Part model, mm, in its own coordinate system. Coordinates: 2 decimals unless noted, no trailing zeros. Order: outer loops, then holes, each group sorted by start corner. A loop starts at its lowest first (then second) coordinate and runs counter-clockwise, first axis right, second up.
from build123d import *

# Parameters (mm, degrees)
F1_DEPTH = 4.253926
F2_R     = 2.54
F3_DEPTH = 4.16477


with BuildPart() as f1:
    # F0 (on Front) → F1 (new body, symmetric)
    with BuildSketch(Plane.XZ):
        Polygon((25.404785, 14.029387), (13.940861, 0), (13.940861, -34.714542), (45.487791, 0), (45.487791, 42.974394), (25.404785, 42.974394), align=None)
    extrude(amount=F1_DEPTH, both=True)

    # F2
    f2_edges = [f1.edges().sort_by_distance(p)[0] for p in [
        (19.672823, -4.253926, 7.014694),
        (13.940861, -4.253926, -17.357271),
        (29.714326, -4.253926, -17.357271),
        (45.487791, -4.253926, 21.487197),
        (35.446288, -4.253926, 42.974394),
        (25.404785, -4.253926, 28.501891),
    ]]
    fillet(f2_edges, radius=F2_R)

    # F1_face (on face) → F3 (join)
    with BuildSketch(Plane(origin=(31.070742, -4.253926, 8.875899), x_dir=(1, 0, 0), z_dir=(0, -1, 0))):
        Polygon((-3.125957, 4.247698), (-14.589881, -9.781689), (-14.589881, -37.01865), (11.87705, -7.894188), (11.87705, 31.558495), (-3.125957, 31.558495), align=None)
    extrude(amount=F3_DEPTH)


solid = f1.part
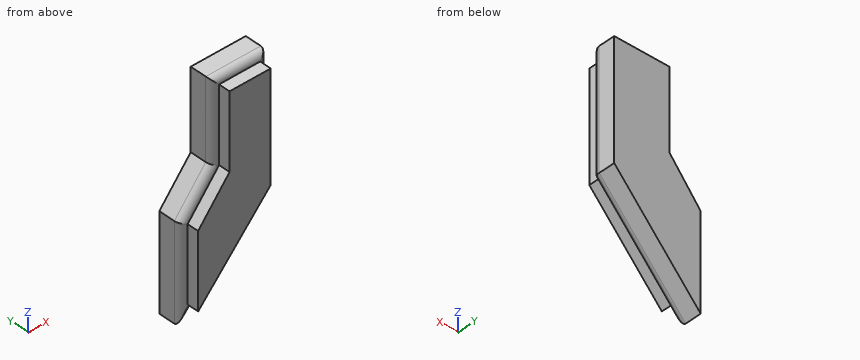
Q1. Pin check, flat tips, straight feed: pin 1 Ø4.5 at (x, y) = (37.5, -7) entering from +Z; pin 2 Ø4 at (x, y) = (21, 0) entering from +Z; pin 3 Ø3.5 at (y, z) = (-7, -19) entering from -X. Stop position of each tip, or through.
Results list:
pin 1: stops at z = 40.43
pin 2: stops at z = 11.09
pin 3: stops at x = 16.48
Q2. Wall check: line 1 along Y through (x, z) = (31.5, -12); line 2 along X through (y, z) = (-1.25, 20.5); line 3 along X through (y, z) = (3.75, -19.5). Give the ranges that are in metal, low to high.
Results list:
line 1: y = -4.24 to 4.25
line 2: x = 25.4 to 45.49
line 3: x = 13.94 to 27.77
Q3. Cut at C-C on y = -0.25. Write the cut outline in (x, z), and give its area (3 significant figures).
Results list:
outline: (13.94, -34.71) - (45.49, 0) - (45.49, 42.97) - (25.4, 42.97) - (25.4, 14.03) - (13.94, 0) - close
area: 1,490 mm2
Q4. Cut at A-A on y = -5.5. Write the cut outline in (x, z), and give its area (3 significant figures).
Results list:
outline: (16.48, -28.14) - (42.95, 0.98) - (42.95, 40.43) - (27.94, 40.43) - (27.94, 13.12) - (16.48, -0.91) - close
area: 1,040 mm2
Q5. Cut at B-B on z = 27.5. Write the cut outline in (x, y), and give its area (3 significant figures).
Results list:
outline: (25.4, -1.71) arc R2.54 ccw to (27.94, -4.25) - (27.94, -8.42) - (42.95, -8.42) - (42.95, -4.25) arc R2.54 ccw to (45.49, -1.71) - (45.49, 4.25) - (25.4, 4.25) - close
area: 231 mm2
